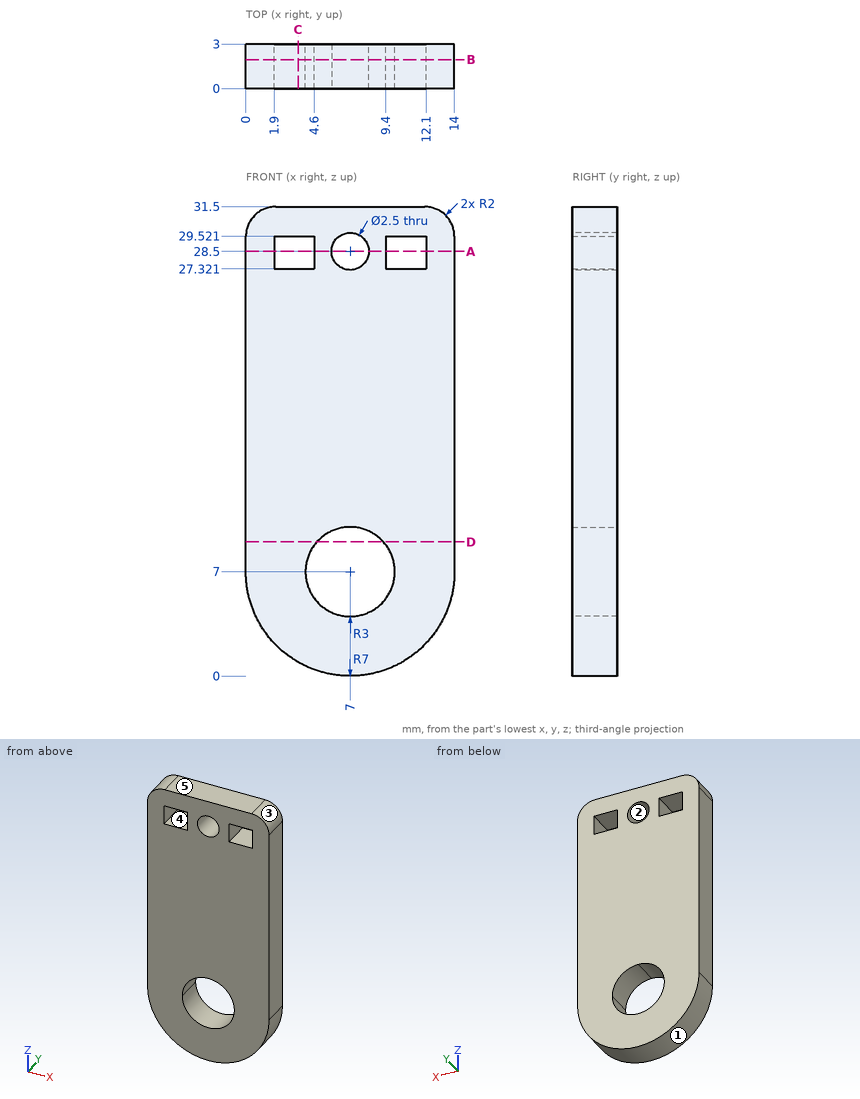
Answer from the drawing. Dimensions are ordinates in mm from the lowest x, y and z of the part. A direction names the side the tool comes from. Round coordinates to 2 decimals unless told otherwise and drop trailing zeros. Write each loop counter-clockwise with the first axis right and the second up, starting at its lowest first coordinate (ties: lowest second). Pieces come first, ordered by that corner, then holes. Notation, with made-up numbers: M 49,51.5 L 101,51.5 A7 cw 101,62.5 Z; hole C 0,-5.75 d9. An arc over 180 degrees is marked long. Write each question's results on one line, items separated by ' | '. Start each with the question number.
Item 1: Which of the six approach directions +Z, -Z, +X, -X, +Y, -Y give full straight-line access (tool end or side, diameter ignored) to the marked faces 4 and 5?
Item 2: Find section D-D on z = 9. Write down the section's boundary in (x, y).
Item 3: Find section A-A on z = 28.5. Write down the section's boundary in (x, y), and give its area (3 significant figures).
Item 4: Straight lines are drawn through the part: probe 1 along X at (y, z) = (1.15, 28.5); probe 2 along Z at (x, y) = (7, 1.55); probe 3 along X at (y, z) = (0.7, 27.5). For each, find the intervals that lie inside material, in ascending order.
Item 5: Find section B-B on y = 1.95. Write down the section's boundary in (x, z), and give its area (3 significant figures).
Item 6: Find section C-C on x = 3.5. Write down the section's boundary in (y, z).
Item 7: The mould has two halves that part along Z. Classify the marked faces 1, 2 and 3: +Z half, -Z half, draft (parallel to the pull), parting line (faces both ways), or undercut.
Item 8: Given pin 1 Ø0.8 at (x, y) = (4, 2) entering from -Z; pin 2 Ø1.5 at (x, z) = (5.5, 23.5) entering from -Y, each flat-ended and moving along its own axis, determine where each tip first touches the part or whether it passes through.
Answer block:
1) face 4: +Y, -Y | face 5: +Z, +X, -X, +Y, -Y
2) outline: M 0,0 L 4.76,0 L 4.76,3 L 0,3 Z; M 9.24,0 L 14,0 L 14,3 L 9.24,3 Z
3) outline: M 0,0 L 1.9,0 L 1.9,3 L 0,3 Z; M 4.6,0 L 5.75,0 L 5.75,3 L 4.6,3 Z; M 8.25,0 L 9.4,0 L 9.4,3 L 8.25,3 Z; M 12.1,0 L 14,0 L 14,3 L 12.1,3 Z | area: 18.3 mm²
4) probe 1: x = 0 to 1.9, 4.6 to 5.75, 8.25 to 9.4, 12.1 to 14 | probe 2: z = 0 to 4, 10 to 27.25, 29.75 to 31.5 | probe 3: x = 0 to 1.9, 4.6 to 6.25, 7.75 to 9.4, 12.1 to 14
5) outline: M 0,7 A7 ccw 14,7 L 14,29.5 A2 ccw 12,31.5 L 2,31.5 A2 ccw 0,29.5 Z; hole M 1.9,27.32 L 4.6,27.32 L 4.6,29.52 L 1.9,29.52 Z; hole C 7,7 d6; hole C 7,28.5 d2.5; hole M 9.4,27.32 L 12.1,27.32 L 12.1,29.52 L 9.4,29.52 Z | area: 373 mm²
6) outline: M 0,0.94 L 3,0.94 L 3,27.32 L 0,27.32 Z; M 0,29.52 L 3,29.52 L 3,31.5 L 0,31.5 Z
7) face 1: -Z half | face 2: undercut | face 3: +Z half
8) pin 1: stops at z = 0.5 | pin 2: stops at y = 0
